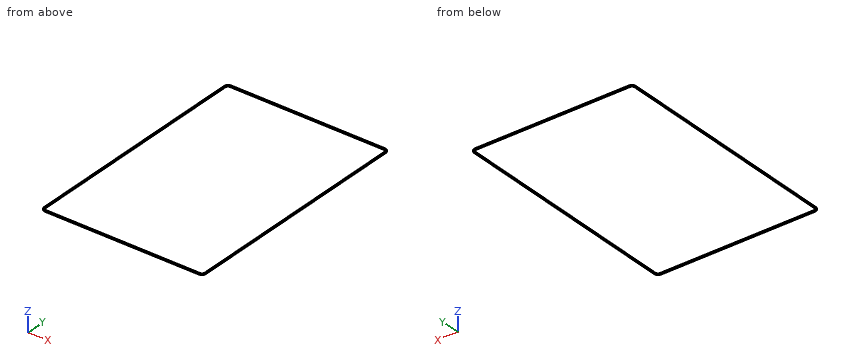
from build123d import *

# Parameters (mm, degrees)
BOSS_EXTRUDE1_DEPTH = 1.778


with BuildPart() as part:
    # Sketch1 → Boss-Extrude1 (new body)
    with BuildSketch(Plane.XY):
        with BuildLine():
            ThreePointArc((4.318, -1.905), (-0.082325499, -0.082325499), (-1.905, 4.318))
            Line((-1.905, 4.318), (-1.905, 385.318))
            ThreePointArc((-1.905, 385.318), (-0.082325499, 389.718325499), (4.318, 391.541))
            Line((4.318, 391.541), (258.318, 391.541))
            ThreePointArc((258.318, 391.541), (262.718325499, 389.718325499), (264.541, 385.318))
            Line((264.541, 385.318), (264.541, 4.318))
            ThreePointArc((264.541, 4.318), (262.718325499, -0.082325499), (258.318, -1.905))
            Line((258.318, -1.905), (4.318, -1.905))
        make_face()
        with BuildLine():
            Line((4.318, -0.127), (258.318, -0.127))
            ThreePointArc((258.318, -0.127), (261.461089642, 1.174910358), (262.763, 4.318))
            Line((262.763, 4.318), (262.763, 385.318))
            ThreePointArc((262.763, 385.318), (261.461089642, 388.461089642), (258.318, 389.763))
            Line((258.318, 389.763), (4.318, 389.763))
            ThreePointArc((4.318, 389.763), (1.174910358, 388.461089642), (-0.127, 385.318))
            Line((-0.127, 385.318), (-0.127, 4.318))
            ThreePointArc((-0.127, 4.318), (1.174910358, 1.174910358), (4.318, -0.127))
        make_face(mode=Mode.SUBTRACT)
    extrude(amount=BOSS_EXTRUDE1_DEPTH)


solid = part.part
Work out the finished part from the listing and answer in its coordinate system (mm). Round coordinates to 2 decimals unless told otherwise and drop trailing zeros. Loops run counter-clockwise (first coordinate to the right, second up) from the corner with the lowest first, then second, coordinate; pieces in that order, holes last. Notation, with made-up numbers: M 10,41 L 35,41 A27 ccw 35,78 Z; hole C 55.5,11.25 d6. An arc over 180 degrees is marked long. One line per question, with ' | ' between items. Start each with the question number.
(1) A cutting plane is placed at A-A on y = 91. Write down the section's boundary in (x, z) (3 decimals), plus the area to 3 significant figures.
(2) A cutting plane is placed at B-B on x = 18.5. Write down the section's boundary in (y, z) (3 decimals).
(3) Find the intervals of material crossed by line 1 (Y direction, x = 226, z = 1.25) (3 decimals); line 2 (X direction, y = 65.5, z = 0.8) (3 decimals), in increasing order.
(4) A cutting plane is placed at C-C on z = 0.95. Write down the section's boundary in (x, y) (3 decimals).
Geometry check:
1) outline: M -1.905,0 L -0.127,0 L -0.127,1.778 L -1.905,1.778 Z; M 262.763,0 L 264.541,0 L 264.541,1.778 L 262.763,1.778 Z | area: 6.32 mm²
2) outline: M -1.905,0 L -0.127,0 L -0.127,1.778 L -1.905,1.778 Z; M 389.763,0 L 391.541,0 L 391.541,1.778 L 389.763,1.778 Z
3) line 1: y = -1.905 to -0.127, 389.763 to 391.541 | line 2: x = -1.905 to -0.127, 262.763 to 264.541
4) outline: M -1.905,4.318 A6.223 ccw 4.318,-1.905 L 258.318,-1.905 A6.223 ccw 264.541,4.318 L 264.541,385.318 A6.223 ccw 258.318,391.541 L 4.318,391.541 A6.223 ccw -1.905,385.318 Z; hole M -0.127,4.318 A4.445 ccw 4.318,-0.127 L 258.318,-0.127 A4.445 ccw 262.763,4.318 L 262.763,385.318 A4.445 ccw 258.318,389.763 L 4.318,389.763 A4.445 ccw -0.127,385.318 Z
